Can you work these out from the model? Positions are in its coordinate system, mm. A direction names the side the tool comes from. Give positions to 0.01 mm unless a question says otherwise; leave off trailing zeros. Write each loop counter-clockwise with the first axis right and the second up, starting at its lowest first coordinate (ties: lowest second). Pieces come first, ordered by that corner, then holes. Notation, with made-up numbers: (28.5, 78.5) - (78.5, 78.5) arc R10 ccw to (78.5, 84.5) - close; hole circle Ø2 at (54.5, -30.5). An arc over 180 degrees is marked (long way). Return JSON: item names as keys, results as strings. Group by question number.
from build123d import *

# Parameters (mm, degrees)
F0_R     = 4.1
F1_DEPTH = 5
F2_W     = 30
F2_H     = 20
F3_DEPTH = 5
F4_R     = 1.55
F4_W     = 10
F4_H     = 5
F5_DEPTH = 5
F6_R     = 2.6
F7_DEPTH = 2.5


with BuildPart() as f1:
    # F0 (on Top) → F1 (new body)
    with BuildSketch(Plane.XY):
        with BuildLine():
            Line((0, 5), (0, 0))
            Line((0, 0), (30, 0))
            Line((30, 0), (30, 5))
            Line((30, 5), (25, 5))
            Line((25, 5), (21, 21))
            ThreePointArc((21, 21), (15, 27), (9, 21))
            Line((9, 21), (5, 5))
            Line((5, 5), (0, 5))
        make_face()
        with BuildLine():
            Line((8.092329, 5), (10.979011, 16.546726))
            ThreePointArc((10.979011, 16.546726), (15, 15), (19.020989, 16.546726))
            Line((19.020989, 16.546726), (21.907671, 5))
            Line((21.907671, 5), (8.092329, 5))
        make_face(mode=Mode.SUBTRACT)
        with Locations((15, 21)):
            Circle(F0_R, mode=Mode.SUBTRACT)
    extrude(amount=F1_DEPTH)

    # F2 (on face) → F3 (join)
    with BuildSketch(Plane.XZ):
        with Locations((15, -5)):
            Rectangle(F2_W, F2_H)
    extrude(amount=-F3_DEPTH)

    # F4 (on face) → F5 (cut)
    with BuildSketch(Plane(origin=(0, 5, 0), x_dir=(-1, 0, 0), z_dir=(0, 1, 0))):
        with Locations((-26.27668, -5)):
            Circle(F4_R)
        with Locations((-3.519477, -5)):
            Circle(F4_R)
        Polygon((-30, -3), (-25, 5), (-30, 5), align=None)
        Polygon((0, -3), (0, 5), (-5, 5), align=None)
        Polygon((-30, -15), (-25, -15), (-30, -7), align=None)
        Polygon((-5, -15), (0, -15), (0, -7), align=None)
        with Locations((-15, -12.5)):
            Rectangle(F4_W, F4_H)
    extrude(amount=-F5_DEPTH, mode=Mode.SUBTRACT)

    # F6 (on face) → F7 (cut)
    with BuildSketch(Plane(origin=(0, 5, 0), x_dir=(-1, 0, 0), z_dir=(0, 1, 0))):
        with Locations((-26.27668, -5)):
            Circle(F6_R)
        with Locations((-3.519477, -5)):
            Circle(F6_R)
    extrude(amount=-F7_DEPTH, mode=Mode.SUBTRACT)


solid = f1.part
1) I need wall thicknesses on line 1 along Y through (x, z) = (15, 3.1); line 2 along Y through (x, z) = (14, 3); line 3 along Z through (x, y) = (8.5, 11.5). Which ranges of each line are inside material? Lowest first, please.
2) Will these pins go through, and if not, where does the flat tip stop? pin 1 Ø5 at (x, z) = (26.28, -5) entering from +Y; pin 2 Ø6 at (x, z) = (26.28, -5) entering from +Y; pin 3 Ø4 at (x, z) = (26, -11) entering from -Y; pin 4 Ø10 at (x, y) = (12.5, 16.5) entering from -Z.
3) Imagine slicing it at A-A, the plane z = -5. Write out the boundary of the cut face in (x, y), and give its area (4 significant figures).
4) Imagine slicing it at B-B, the plane x = 15. Write out the boundary of the cut face in (y, z), and give its area (3 significant figures).
5) On a 3-axis mill with a long thin cutter (end or side, diameter ignored), from which of +Z, -Z, +X, -X, +Y, -Y can I reach the whole of each face in a straight line? I mean faces 1 (the face through (14, 16, 0)), 2 (the face through (27.535, 2.535, 0.944)), 3 (the face through (20, 3, -13)), 4 (the face through (23.797, 3.768, -4.219)). Say none if no direction works.
6) Imagine slicing it at C-C, the plane y = 19.25. Write out the boundary of the cut face in (x, z), and give its area (3 significant figures).
7) Imagine slicing it at D-D, the plane x = 3.5. Write out the boundary of the cut face in (y, z).
8) We'd pull the mould along Z, two halves only. Please class faces 5 (the face through (22, 2, -15)), 6 (the face through (1.04, 3.77, -4.22)), 7 (the face through (30, 2, -5)), 8 (the face through (26, 2.5, -7)): pulls with the +Z half, pulls with the -Z half, needs draft (parallel to the pull), parting line crosses it, or undercut.
Resolved:
{
 "1": {"line 1": "0 to 5, 15 to 16.9, 25.1 to 27", "line 2": "0 to 5, 15.08 to 17.02, 24.98 to 26.92", "line 3": "0 to 5"},
 "2": {"pin 1": "y = 2.5", "pin 2": "y = 5", "pin 3": "y = 0", "pin 4": "z = 0"},
 "3": {"outline": "(0, 0) - (1.97, 0) - (1.97, 2.5) - (0.92, 2.5) - (0.92, 5) - (0, 5) - close; (5.07, 0) - (24.73, 0) - (24.73, 2.5) - (23.68, 2.5) - (23.68, 5) - (6.12, 5) - (6.12, 2.5) - (5.07, 2.5) - close; (27.83, 0) - (30, 0) - (30, 5) - (28.88, 5) - (28.88, 2.5) - (27.83, 2.5) - close", "area": "108.5 mm^2"},
 "4": {"outline": "(0, -10) - (5, -10) - (5, 5) - (0, 5) - close; (15, 0) - (16.9, 0) - (16.9, 5) - (15, 5) - close; (25.1, 0) - (27, 0) - (27, 5) - (25.1, 5) - close", "area": "94.0 mm^2"},
 "5": {"face 1": "-Z, +X, -X, +Y", "face 2": "+Z, +X, +Y, -Y", "face 3": "-Z, +Y, -Y", "face 4": "+Y"},
 "6": {"outline": "(8.56, 0) - (11.29, 0) - (11.29, 5) - (8.56, 5) - close; (18.71, 0) - (21.44, 0) - (21.44, 5) - (18.71, 5) - close", "area": "27.3 mm^2"},
 "7": {"outline": "(0, -12.6) - (5, -12.6) - (5, -7.6) - (2.5, -7.6) - (2.5, -6.55) - (0, -6.55) - close; (0, -3.45) - (2.5, -3.45) - (2.5, -2.4) - (5, -2.4) - (5, 2.6) - (0, 2.6) - close"},
 "8": {"face 5": "pulls with the -Z half", "face 6": "undercut", "face 7": "needs draft", "face 8": "undercut"}
}
